For this review, take the finished solid that the model builds, in its own axes (mm). A direction names the side the tool comes from. Coordinates: 2 decimals unless noted, no trailing zeros. Order: outer loops, then holes, each group sorted by start corner. A loop starts at its lowest first (then second) coordinate and runs counter-clockwise, first axis right, second up.
from build123d import *

# Parameters (mm, degrees)
F0_R     = 40.248504
F1_DEPTH = 101.6
F2_R     = 26.250154
F3_DEPTH = 7.62
F4_R     = 5.08
F5_R     = 5.08


with BuildPart() as f1:
    # F0 (on Top) → F1 (new body)
    with BuildSketch(Plane.XY):
        Circle(F0_R)
    extrude(amount=F1_DEPTH)

    # F2 (on face) → F3 (join)
    with BuildSketch(Plane.XY.offset(101.6)):
        Circle(F2_R)
    extrude(amount=F3_DEPTH)

    # F4
    f4_edges = [f1.edges().sort_by_distance(p)[0] for p in [
        (-26.250154, 0, 109.22),
    ]]
    fillet(f4_edges, radius=F4_R)

    # F5
    f5_edges = [f1.edges().sort_by_distance(p)[0] for p in [
        (-40.248504, 0, 101.6),
    ]]
    fillet(f5_edges, radius=F5_R)


solid = f1.part
1. To check wall thickness, follow L1, parallel to Z at x = -32.5, y = -1.5; L2, parallel to Y at x = -26, z = 13.5; L3, parallel to Y at x = 34.5, z = 83. State the ranges of each line that lie inside material, in increasing order.
Answer below:
L1: z = 0 to 101.6
L2: y = -30.72 to 30.72
L3: y = -20.73 to 20.73
2. Take a section at C-C, the plane z = 26.5. Give the boundary of the cut face in (x, y).
Answer below:
outline: circle Ø80.5 at (0, 0)
3. Machinability: for faces 1 (the face through (0, 0, 109.22)), 2 (the face through (-5.691, -25.626, 102.852)), which of the approach directions +Z, -Z, +X, -X, +Y, -Y give a long, thin tool a straight path to every point of the face, cutting with its end or side? Answer none if there is none.
Answer below:
face 1: +Z, +X, -X, +Y, -Y
face 2: +Z
4. Take a section at A-A, the plane x = 0. Give the boundary of the cut face in (y, z), plus the area to 3 significant figures.
Answer below:
outline: (-40.25, 0) - (40.25, 0) - (40.25, 96.52) arc R5.08 ccw to (35.17, 101.6) - (26.25, 101.6) - (26.25, 104.14) arc R5.08 ccw to (21.17, 109.22) - (-21.17, 109.22) arc R5.08 ccw to (-26.25, 104.14) - (-26.25, 101.6) - (-35.17, 101.6) arc R5.08 ccw to (-40.25, 96.52) - close
area: 8,560 mm2
5. Clearance check with flat-ended pins moving along their axes: pin 1 Ø10 at (y, z) = (15.5, 15) entering from -X; pin 2 Ø5 at (x, z) = (-7, 78) entering from +Y; pin 3 Ø1.5 at (x, y) = (1, -32) entering from +Z. State where each tip first meets the part, or that it passes through.
Answer below:
pin 1: stops at x = -38.85
pin 2: stops at y = 40
pin 3: stops at z = 101.6
